```python
from build123d import *

# Parameters (mm, degrees)
BOSS_EXTRUDE1_DEPTH    = 11
SKETCH2_W              = 2
SKETCH2_H              = 6
BOSS_EXTRUDE2_DEPTH    = 2
SKETCH1_3_W            = 2
SKETCH1_3_H            = 100
BOSS_EXTRUDE3_DEPTH    = 11
SKETCH3_W              = 12
SKETCH3_H              = 100
BOSS_EXTRUDE4_DEPTH    = 2
SKETCH10_W             = 12
SKETCH10_H             = 28.85
CUT_EXTRUDE3_DEPTH     = 14
SKETCH11_W             = 12
SKETCH11_H             = 13
BOSS_EXTRUDE8_DEPTH    = 2
SKETCH12_W             = 8
SKETCH12_H             = 11
CUT_EXTRUDE4_DEPTH     = 2
SKETCH17_W             = 13
SKETCH17_H             = 16.3
CUT_EXTRUDE7_DEPTH     = 26.8
SKETCH18_W             = 11
SKETCH18_H             = 6
BOSS_EXTRUDE11_DEPTH   = 2
SKETCH19_W             = 8
SKETCH19_H             = 11
BOSS_EXTRUDE12_DEPTH   = 2
FILLET8_R              = 2
SKETCH20_W             = 0.5
SKETCH20_H             = 4
BOSS_EXTRUDE13_DEPTH   = 5.8
BOSS_EXTRUDE13_2_DEPTH = 5.8
BOSS_EXTRUDE14_DEPTH   = 4


with BuildPart() as part:
    # Sketch1 → Boss-Extrude1 (new body)
    with BuildSketch(Plane.XY):
        Polygon((24.8, 14.3), (-2, 14.3), (-2, -2), (24.8, -2), (24.8, 3.15), (22.8, 3.15), (22.8, 0), (0, 0), (0, 12.3), (22.8, 12.3), (22.8, 9.15), (24.8, 9.15), align=None)
    extrude(amount=BOSS_EXTRUDE1_DEPTH)

    # Sketch2 → Boss-Extrude2 (add)
    with BuildSketch(Plane.XY.offset(11)):
        Polygon((22.8, 9.15), (22.8, 3.15), (22.8, 0), (0, 0), (0, 12.3), (22.8, 12.3), align=None)
        Polygon((24.8, -2), (24.8, 3.15), (22.8, 3.15), (22.8, 0), (0, 0), (0, 12.3), (22.8, 12.3), (22.8, 9.15), (24.8, 9.15), (24.8, 14.3), (-2, 14.3), (-2, -2), align=None)
        with Locations((23.8, 6.15)):
            Rectangle(SKETCH2_W, SKETCH2_H)
    extrude(amount=BOSS_EXTRUDE2_DEPTH)

    # Sketch1_3 → Boss-Extrude3 (add)
    with BuildSketch(Plane.XY):
        Polygon((24.8, 3.15), (24.8, -2), (24.8, -43.85), (26.8, -43.85), (26.8, 3.15), align=None)
        Polygon((24.8, 56.15), (24.8, 14.3), (24.8, 9.15), (26.8, 9.15), (26.8, 56.15), align=None)
        with Locations((35.8, 6.15)):
            Rectangle(SKETCH1_3_W, SKETCH1_3_H)
    extrude(amount=BOSS_EXTRUDE3_DEPTH)

    # Sketch3 → Boss-Extrude4 (add)
    with BuildSketch(Plane.XY.offset(11)):
        with Locations((30.8, 6.15)):
            Rectangle(SKETCH3_W, SKETCH3_H)
    extrude(amount=BOSS_EXTRUDE4_DEPTH)

    # Sketch10 → Cut-Extrude3 (cut, through all)
    with BuildSketch(Plane.XY.offset(13)):
        with Locations((30.8, 41.725)):
            Rectangle(SKETCH10_W, SKETCH10_H)
    extrude(amount=-CUT_EXTRUDE3_DEPTH, mode=Mode.SUBTRACT)

    # Sketch11 → Boss-Extrude8 (add)
    with BuildSketch(Plane(origin=(0, 27.3, 0), x_dir=(1, 0, 0), z_dir=(0, 1, 0))):
        with Locations((30.8, -6.5)):
            Rectangle(SKETCH11_W, SKETCH11_H)
    extrude(amount=-BOSS_EXTRUDE8_DEPTH)

    # Sketch12 → Cut-Extrude4 (cut)
    with BuildSketch(Plane.XY.offset(13)):
        with Locations((30.8, 19.8)):
            Rectangle(SKETCH12_W, SKETCH12_H)
    extrude(amount=-CUT_EXTRUDE4_DEPTH, mode=Mode.SUBTRACT)

    # Sketch17 → Cut-Extrude7 (cut)
    with BuildSketch(Plane.ZY.offset(2)):
        with Locations((6.5, 6.15)):
            Rectangle(SKETCH17_W, SKETCH17_H)
    extrude(amount=-CUT_EXTRUDE7_DEPTH, mode=Mode.SUBTRACT)

    # Sketch18 → Boss-Extrude11 (add)
    with BuildSketch(Plane.ZY.offset(-24.8)):
        with Locations((5.5, 6.15)):
            Rectangle(SKETCH18_W, SKETCH18_H)
    extrude(amount=-BOSS_EXTRUDE11_DEPTH)

    # Sketch19 → Boss-Extrude12 (add)
    with BuildSketch(Plane.XY.offset(13)):
        with Locations((30.8, 19.8)):
            Rectangle(SKETCH19_W, SKETCH19_H)
    extrude(amount=-BOSS_EXTRUDE12_DEPTH)

    # Fillet8
    fillet8_edges = [part.edges().sort_by_distance(p)[0] for p in [
        (36.8, 27.3, 6.5),
        (24.8, 27.3, 6.5),
        (30.8, 27.3, 13),
        (24.8, -8.275, 13),
        (36.8, -8.275, 13),
    ]]
    fillet(fillet8_edges, radius=FILLET8_R)



with BuildPart() as body_2:
    # Sketch20 → Boss-Extrude13 (new body)
    with BuildSketch(Plane(origin=(0, 0, 0), x_dir=(-1, 0, 0), z_dir=(0, 0, -1))):
        with Locations((-34.55, 22.3)):
            Rectangle(SKETCH20_W, SKETCH20_H)
    extrude(amount=BOSS_EXTRUDE13_DEPTH)


with BuildPart() as body_3:
    # Sketch20 → Boss-Extrude13 2 (new body)
    with BuildSketch(Plane(origin=(0, 0, 0), x_dir=(-1, 0, 0), z_dir=(0, 0, -1))):
        with Locations((-27.05, 22.3)):
            Rectangle(SKETCH20_W, SKETCH20_H)
    extrude(amount=BOSS_EXTRUDE13_2_DEPTH)


with BuildPart() as part_1:
    add(part.part)

    add(body_2.part)  # Boss-Extrude14 merges body 2

    add(body_3.part)  # Boss-Extrude14 merges body 3
    # Sketch21 → Boss-Extrude14 (add)
    with BuildSketch(Plane.XZ.offset(-20.3)):
        Polygon((27.3, 0.5), (26.8, 1), (26.8, 0.5), (26.8, 0), (27.3, 0), align=None)
        Polygon((26.8, -5.8), (25.8, -5.8), (27.05, -7.3), (27.3, -7.3), (27.3, -5.8), align=None)
        Polygon((34.3, -5.8), (34.8, -5.8), (35.8, -5.8), (34.55, -7.3), (34.3, -7.3), align=None)
        Polygon((34.8, 0), (34.3, 0), (34.3, 0.5), (34.8, 1), (34.8, 0.5), align=None)
    extrude(amount=-BOSS_EXTRUDE14_DEPTH)


solid = part_1.part
```
Can you work these out from the model? Positions are in its coordinate system, mm. A direction names the side the tool comes from. Coordinates: 2 decimals unless noted, no trailing zeros. Order: outer loops, then holes, each group sorted by start corner. A loop starts at its lowest first (then second) coordinate and runs counter-clockwise, first axis right, second up.
1. If we section it at C-C (x = 29.5): Please give me the cut outline in (y, z).
2. If we section it at A-A (z = -4): Please give me the cut outline in (x, y).
3. If we section it at D-D (z = 9.25): Please give me the cut outline in (x, y), then the cut area to 3 significant figures.
4. For faces 1 (the face through (31, 27.3, 6)), 2 (the face through (26.8, 22, -3)), which set-ups out of +Z, -Z, +X, -X, +Y, -Y let a thin tool reach every point of the face, with its end or its side?
5. I need wall thicknesses on line 1 (X direction, y = -16, z = 10.75); line 2 (Y direction, x = 29.75, z = 4.75); line 3 (Z direction, x = 29.5, y = -28.5). Which ranges of each line are inside material? Lowest first, please.
6. If we section it at B-B (y = 18.5): Please give me the cut outline in (x, z).
7. I'm going to push flat-ended pins straight in: pin 1 (3.5 mm diameter, centred on x = 31.5, y = 3, fed in from -Z); pin 2 (1.6 mm diameter, centred on x = 35.5, z = -2, fed in from +Y); pin 3 (3 mm diameter, centred on y = 23, z = -2, fed in from +X); pin 4 (6 mm diameter, centred on x = 31, z = -4.5, fed in from -Y). Where does each tip first touch, or does it pass through?
8. Thinking about a two-plate mould opening in X: for faces 3 (the face through (31, 25.3, 5)), 4 (the face through (26, -6, 0)), 5 (the face through (25.4, -8.79, 12.43)), which applies, +X half, -X half, draft (parallel to the pull), parting line (faces both ways), or undercut?
Entries:
1. outline: (-43.85, 11) - (25.3, 11) - (25.3, 0) - (27.3, 0) - (27.3, 11) arc R2 ccw to (25.3, 13) - (-43.85, 13) - close
2. outline: (26.8, 20.3) - (27.3, 20.3) - (27.3, 24.3) - (26.8, 24.3) - close; (34.3, 20.3) - (34.8, 20.3) - (34.8, 24.3) - (34.3, 24.3) - close
3. outline: (24.8, -43.85) - (26.8, -43.85) - (26.8, 25.3) - (34.8, 25.3) - (34.8, -43.85) - (36.8, -43.85) - (36.8, 25.3) arc R2 ccw to (34.8, 27.3) - (26.8, 27.3) arc R2 ccw to (24.8, 25.3) - close
3. area: 299 mm2
4. face 1: +Z, -Z, +X, -X, +Y
4. face 2: -X, +Y, -Y
5. line 1: x = 24.8 to 26.8, 34.8 to 36.8
5. line 2: y = 25.3 to 27.3
5. line 3: z = 11 to 13
6. outline: (24.8, 0) - (26.8, 0) - (26.8, 11) - (34.8, 11) - (34.8, 0) - (36.8, 0) - (36.8, 11) arc R2 ccw to (34.8, 13) - (26.8, 13) arc R2 ccw to (24.8, 11) - close
7. pin 1: stops at z = 11
7. pin 2: stops at y = 24.3
7. pin 3: stops at x = 34.8
7. pin 4: passes through
8. face 3: undercut
8. face 4: draft
8. face 5: -X half
